Solid Edge part; units mm, degrees
sketch "Sketch1" plane through (0, 0, 0) normal (0, -1, 0) x (1, 0, 0)
  line L0 (3.5, 4) -> (3.5, 0)
  line L1 (3.5, 0) -> (2.35, 0)
  line L2 (2.35, 0) -> (2, -0.6062)
  line L3 (2, -0.6062) -> (2, -12)
  line L4 (2, -12) -> (0, -12)
  line L5 (1.5, 2) -> (0, 1.834)
  line L6 (1.5, 4) -> (1.5, 2)
  line L7 (3.5, 4) -> (1.5, 4)
revolve "RevolvedProtrusion1" add sketch "Sketch1" angle 360 about axis through (0, 0, -6) along (0, 0, 1)
cosmetic_thread "Thread1"
chamfer "mounting_chamfer" distance 0.4 angle 45 1 edges at (-2, 0, -12)
fillet "head_round" radius 0.4 2 edges at (-3.5, 0, 0) (-3.5, 0, 4)
sketch "Sketch2" plane through (0, 0, 4) normal (0, 0, 1) x (0, 1, 0)
  line L0 (-1.5, 0.866) -> (-1.5, -0.866)
  line L1 (0, -1.7321) -> (-1.5, -0.866)
  line L2 (1.5, -0.866) -> (0, -1.7321)
  line L3 (1.5, 0.866) -> (1.5, -0.866)
  line L4 (0, 1.7321) -> (1.5, 0.866)
  line L5 (-1.5, 0.866) -> (0, 1.7321)
extrude "Cutout1" cut sketch "Sketch2" against normal up to vertex (2 mm away)
properties part number "STD-DIN912-M4x12" material "Galvanized steel"
Could you check a few things on this model? Use its own coordinates, in mm. A direction names the side the tool comes from. Give positions to 0.01 mm unless a question says otherwise; leave off trailing zeros. Order: outer loops, then holes, each group sorted by start corner. A loop starts at its lowest first (then second) coordinate and runs counter-clockwise, first axis right, second up.
Q1. We'd pull the mould along X, two halves only. Please class faces 4 (the cylindrical face through (0, 2, -6)), 5 (the flat face through (0, 0, -12)), 6 (the flat face through (-1.293, -0.76, 3.014)): +X half, -X half, draft (parallel to the pull), parting line (faces both ways), or undercut.
Q2. I'm going to push flat-ended pins straight in: P1, Ø1.5, axis at x = 2, z = 0.5, coming from the -Y side; P2, Ø2, axis at y = 1, z = -3.5, coming from the -X side; P3, Ø2, axis at y = 2, z = -2, coming from the +X side. Where does each tip first touch, or does it pass through?
Q3. Suppose I cut it at A-A, the plane z = -10. Write out the boundary of the cut face in (x, y), and give its area (3 significant figures).
Q4. For faces 1 (the flat face through (-1.305, 0.74, 3.014)), 2 (the flat face through (-2, 2, 0)), 3 (the cylindrical face through (3.233, 1.341, 1.978)), which set-ups out of +Z, -Z, +X, -X, +Y, -Y let a thin tool reach every point of the face, with its end or its side?
Q5. Suppose I cut it at B-B, the plane z = 1. Write out the boundary of the cut face in (x, y), and give its area (3 significant figures).
Q6. If I drill on line 1 along Z through (x, y) = (0, 2.75); line 2 along X through (y, z) = (-0.25, 3.25); line 3 along Y through (x, z) = (-1, -3), over which ranges is the centre line in solid material (lowest first)?
Solution:
1. face 4: parting line
1. face 5: draft
1. face 6: undercut
2. P1: stops at y = -3.27
2. P2: stops at x = -2
2. P3: stops at x = 1.73
3. outline: circle Ø4 at (0, 0)
3. area: 12.6 mm2
4. face 1: +Z
4. face 2: -Z
4. face 3: +Z, -Z
5. outline: circle Ø7 at (0, 0)
5. area: 38.5 mm2
6. line 1: z = 0 to 4
6. line 2: x = -3.49 to -1.59, 1.59 to 3.49
6. line 3: y = -1.73 to 1.73
